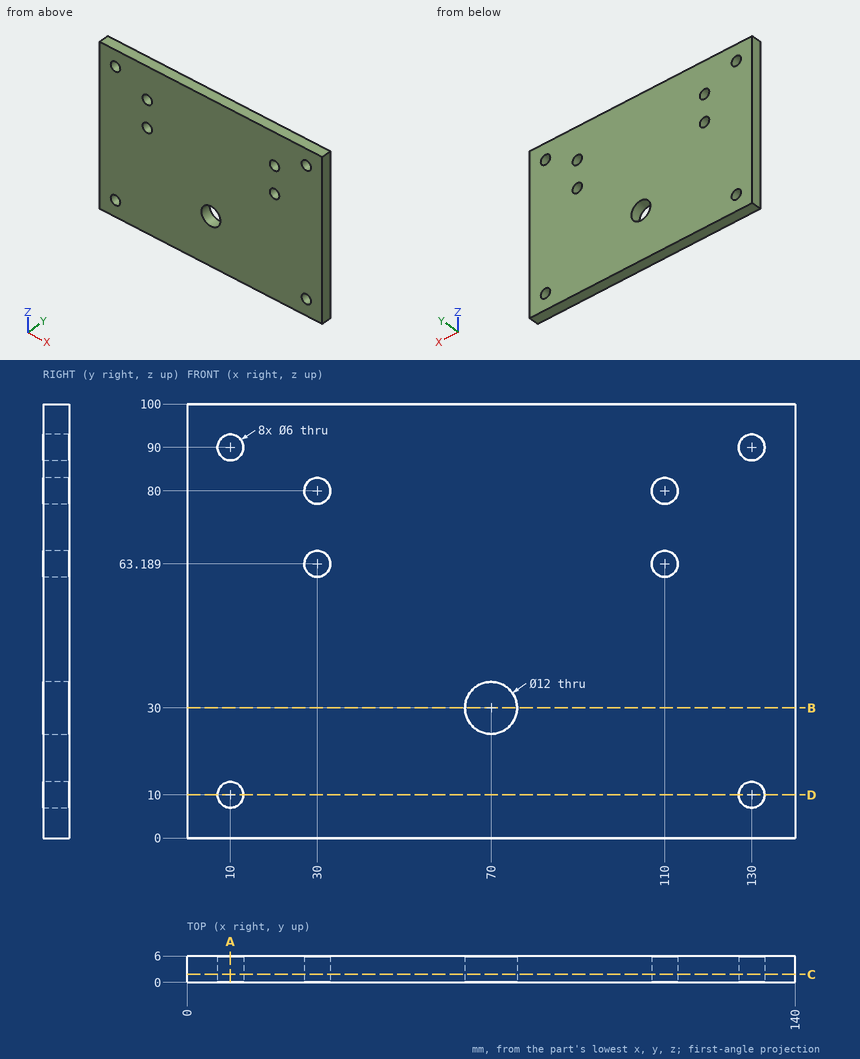
Job drawing, mm, ordinate dimensions from the low corner. One solid piece. Round coordinates to 2 decimals unless told otherwise and drop trailing zeros. Write each loop counter-clockwise with the first axis right and the second up, starting at its lowest first coordinate (ties: lowest second). Pieces come first, ordered by that corner, then holes.
1) Band-saw the part on D-D, the plane z = 10. List the corners of the cut face in (x, y).
2) Band-saw the part on B-B, the plane z = 30. List the corners of the cut face in (x, y).
3) Drill centre lines: probe 1 along Z at (x, y) = (110, 3.25); probe 2 along X at (y, z) = (3.95, 80); probe 3 along X at (y, z) = (2.6, 90). Where is each one in solid material? Low to high.
4) Band-saw the part on A-A, the plane x = 10. List the corners of the cut face in (y, z).
5) Band-saw the part on C-C, the plane y = 1.8. Give the number of separate pieces and of enclosed holes in the cut face, and give its area (3 significant figures).
Ans:
1. outline: (0, 0) - (7, 0) - (7, 6) - (0, 6) - close; (13, 0) - (127, 0) - (127, 6) - (13, 6) - close; (133, 0) - (140, 0) - (140, 6) - (133, 6) - close
2. outline: (0, 0) - (64, 0) - (64, 6) - (0, 6) - close; (76, 0) - (140, 0) - (140, 6) - (76, 6) - close
3. probe 1: z = 0 to 60.19, 66.19 to 77, 83 to 100
3. probe 2: x = 0 to 27, 33 to 107, 113 to 140
3. probe 3: x = 0 to 7, 13 to 127, 133 to 140
4. outline: (0, 0) - (6, 0) - (6, 7) - (0, 7) - close; (0, 13) - (6, 13) - (6, 87) - (0, 87) - close; (0, 93) - (6, 93) - (6, 100) - (0, 100) - close
5. separate pieces: 1
5. enclosed holes: 9
5. area: 13,700 mm2
